from build123d import *

# Parameters (mm, degrees)
SKETCH1_R           = 5.5
BOSS_EXTRUDE1_DEPTH = 160
SKETCH2_W           = 11
SKETCH2_H           = 11
BOSS_EXTRUDE2_DEPTH = 10
BOSS_EXTRUDE3_DEPTH = 20
CIRPATTERN1_COUNT   = 2
SKETCH4_R           = 1.625
CUT_EXTRUDE1_DEPTH  = 45


with BuildPart() as part:
    # Sketch1 → Boss-Extrude1 (new body)
    with BuildSketch(Plane(origin=(0, 0, 0), x_dir=(1, 0, 0), z_dir=(0, 1, 0))):
        with Locations(Location((0, 0, 0), (0, 0, 270))):
            Circle(SKETCH1_R)
    extrude(amount=BOSS_EXTRUDE1_DEPTH)

    # Sketch2 → Boss-Extrude2 (add)
    with BuildSketch(Plane(origin=(0, 160, 0), x_dir=(1, 0, 0), z_dir=(0, 1, 0))):
        Rectangle(SKETCH2_W, SKETCH2_H)
    extrude(amount=BOSS_EXTRUDE2_DEPTH)

    # Sketch3 → Boss-Extrude3 (add)
    with BuildSketch(Plane.ZY.offset(5.5)):
        Polygon((-5.386751346, 170), (-0.386751346, 170), (5.386751346, 160), (0.386751346, 160), align=None)
    boss_extrude3 = extrude(amount=BOSS_EXTRUDE3_DEPTH)

    # CirPattern1: Boss-Extrude3 ×2 about axis
    cirpattern1_axis = Axis((0, 0, 0), (0, 1, 0))
    for i in range(1, CIRPATTERN1_COUNT):
        add(boss_extrude3.rotate(cirpattern1_axis, i * 360 / CIRPATTERN1_COUNT))

    # Sketch4 → Cut-Extrude1 (cut)
    with BuildSketch(Plane.XZ):
        with Locations(Location((0, 0, 0), (0, 0, 270))):
            Circle(SKETCH4_R)
    extrude(amount=-CUT_EXTRUDE1_DEPTH, mode=Mode.SUBTRACT)


solid = part.part
Model file for the job. Use its own axes, mm. A direction names the side the tool comes from. Give positions to 0.01 mm unless a question says otherwise; leave off trailing zeros. Order: outer loops, then holes, each group sorted by start corner. A loop starts at its lowest first (then second) coordinate and runs counter-clockwise, first axis right, second up. Notation, with made-up numbers: (16, 20.5) -> (61, 20.5) arc R24 ccw to (61, 51.5) -> close; hole circle Ø10 at (40.25, 8). An arc over 180 degrees is marked (long way). Use CSV: the item, a comma, the result in double quotes.
1. Band-saw the part on B-B, the plane x = -16.5. Give the cut face in (y, z), then the cut area to 3 significant figures.
Outcome:
outline,"(160, 0.39) -> (170, -5.39) -> (170, -0.39) -> (160, 5.39) -> close"
area,"50.0 mm²"
2. Drop flat-ended pins along their axis: pin 1 (1.6 mm diameter, centred on x = 0.5, z = 0.5, fed in from -Y); pin 2 (1 mm diameter, centred on y = 122.5, z = -1.5, fed in from -X); pin 3 (6 mm diameter, centred on x = -12.5, z = 2.5, fed in from -Y). Give the stop position or say it passes through.
Outcome:
pin 1,"y = 45"
pin 2,"x = -5.41"
pin 3,"y = 160"
3. Band-saw the part on A-A, the plane y = 151. Give the cut face in (x, z).
Outcome:
outline,"circle Ø11 at (0, 0)"
4. Mould opens along X. For faces 1 (the flat face through (15.36, 164.93, 2.46)), 2 (the cylindrical face through (-5.37, 78.88, -1.19)), 3 (the flat face through (-5.5, 164, -3)), 4 (the flat face through (0, 45, 0)) say: +X half, -X half, draft (parallel to the pull), parting line (faces both ways), or undercut.
Outcome:
face 1,"draft"
face 2,"parting line"
face 3,"-X half"
face 4,"undercut"
5. Drill centre lines: line 1 along X through (y, z) = (145, 1.25); line 2 along Y through (x, z) = (-1, 0); line 3 along Y through (x, z) = (7, 0). Where is each one in solid material? Low to high. Write a range as from..to.
Outcome:
line 1,"-5.36..5.36"
line 2,"45..170"
line 3,"160.67..169.33"
6. 3-axis set-ups, long thin cutter, end or side, ignore diameter. For faces 5 (the flat face through (4, 160, 4)), 6 (the cylindrical face through (-0.99, 22.18, 1.29)), 7 (the flat face through (-4, 160, -4)), 8 (the flat face through (15.36, 165.07, -2.46)), 9 (the flat face through (-5.5, 166, 3)): which of +Z, -Z, +X, -X, +Y, -Y reach the whole face in a straight line?
Outcome:
face 5,"+Z, +X, -Y"
face 6,"-Y"
face 7,"-Z, -X, -Y"
face 8,"-Z, +X, +Y"
face 9,"+Z, -X, +Y"
